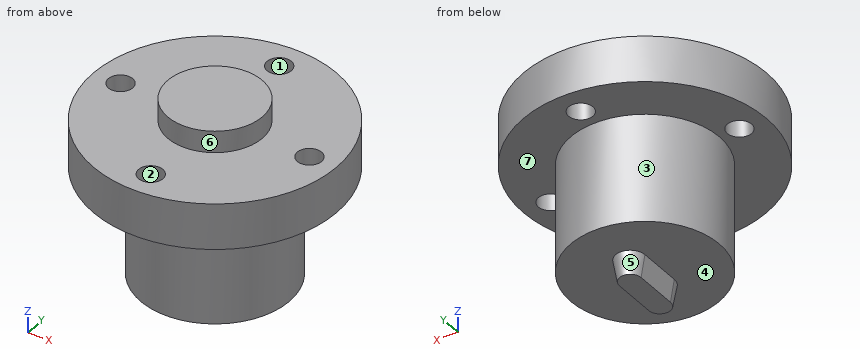
Autodesk Inventor part; units mm, degrees
ref_plane "YZ Plane" through (0, 0, 0) normal (1, 0, 0) x (0, 1, 0)
ref_plane "XZ Plane" through (0, 0, 0) normal (0, 1, 0) x (-1, 0, 0)
ref_plane "XY Plane" through (0, 0, 0) normal (0, 0, 1) x (1, 0, 0)
sketch "Esboço1" plane through (0, 0, 0) normal (0, 0, 1) x (1, 0, 0)
  circle A0 centre (0, 0) radius 27.5
  dimension "d0" = 55
extrude "Extrusão1" add sketch "Esboço1" along normal blind 40
sketch "Esboço2" plane through (0, 0, 40) normal (0, 0, 1) x (1, 0, 0)
  circle A0 centre (0, 0) radius 45
  dimension "d3" = 90
extrude "Extrusão2" add sketch "Esboço2" along normal blind 17
sketch "Esboço3" plane through (0, 0, 57) normal (0, 0, 1) x (1, 0, 0)
  circle A0 centre (35, 0) radius 4.5
  circle A1 centre (0, 35) radius 4.5
  circle A2 centre (-35, 0) radius 4.5
  circle A3 centre (0, -35) radius 4.5
  point P0 (0, 0)
  dimension "d7" = 9
  dimension "d8" = 35
  dimension "d11" = 360
extrude "Extrusão3" cut sketch "Esboço3" against normal blind 17.5
sketch "Esboço4" plane through (0, 0, 57) normal (0, 0, 1) x (1, 0, 0)
  circle A0 centre (0, 0) radius 27.5
  circle A1 centre (0, 0) radius 17.5
  dimension "d15" = 35
extrude "Extrusão4" add sketch "Esboço4" along normal blind 8 contours A1
sketch "Esboço6" plane through (0, 0, 0) normal (0, 0, -1) x (-1, 0, 0)
  line L0 (0, 8) -> (0, -8) construction
  line L1 (5.41, 8) -> (5.41, -8)
  line L2 (-5.41, -8) -> (-5.41, 8)
  arc A0 (5.41, 8) -> (-5.41, 8) centre (0, 8) ccw
  arc A1 (-5.41, -8) -> (5.41, -8) centre (0, -8) ccw
  point P0 (0, 0)
  point P1 (0, 0)
  dimension "d24" = 5.41
  dimension "d25" = 16
  dimension "d26" = 0
  dimension "d27" = 0
extrude "Extrusão5" add sketch "Esboço6" along normal blind 8 draft -10
properties part number "Matriz superior do Ferramental"
Verification items for the finished model (mm, model axes). Face numbers are marked on the shaded views. A direction names the side the tool comes from. Give positions to 0.01 mm unless a question says otherwise; leave off trailing zeros. Order: outer loops, then holes, each group sorted by start corner. A loop starts at its lowest first (then second) coordinate and runs counter-clockwise, first axis right, second up. Notation, with made-up numbers: M -22,56.25 L 0,56.25 A18 ccw 0,81.25 Z; hole C 67.5,-2.75 d9. An arc over 180 degrees is marked long. Return JSON: item names as keys, results as strings. Group by question number.
1) Section check B-B on x = 36. Record the cut outline in (y, z), and give its area (3 significant figures).
2) Section check C-C on x = 0. Record the cut outline in (y, z), and give its area (3 significant figures).
3) Go/stop test with flat-tipped pins: pin 1 Ø2 at (x, z) = (19.5, 9.5) entering from +Y; pin 2 Ø14.5 at (x, y) = (0, -35) entering from +Z; pin 3 Ø2 at (x, z) = (-17, 26.5) entering from -Y. Record where each tip stops, or that it passes through.
4) Section check D-D on z = 53. Record the cut outline in (x, y).
5) Section check A-A on y = 0. Record the cut outline in (x, z), and give its area (3 significant figures).
6) Mould release check, pull along Y, two halves, no side actions. Record for the marked faces 1, 2, 3 and 4: pulls with the +Y half, pulls with the -Y half, needs draft (parallel to the pull), parting line crosses it, or undercut.
7) Access from +Z, -Z, +X, -X, +Y, -Y to the whole of each face (thin tool, end or side, straight path). Record for the marked faces 5, 6 and 7.
8) Scan lines: line 1 (Y direction, x = 0, z = 49); line 2 (Z direction, x = 34, y = 23.5); line 3 (X direction, y = -2, z = 55). Record each from-to range of solid material in increasing order.
Answer block:
{
 "1": {"outline": "M -27,40 L -4.39,40 L -4.39,57 L -27,57 Z; M 4.39,40 L 27,40 L 27,57 L 4.39,57 Z", "area": "769 mm^2"},
 "2": {"outline": "M -45,40 L -39.5,40 L -39.5,57 L -45,57 Z; M -30.5,40 L -27.5,40 L -27.5,0 L -13.41,0 L -12,-8 L 12,-8 L 13.41,0 L 27.5,0 L 27.5,40 L 30.5,40 L 30.5,57 L 17.5,57 L 17.5,65 L -17.5,65 L -17.5,57 L -30.5,57 Z; M 39.5,40 L 45,40 L 45,57 L 39.5,57 Z", "area": "3,910 mm^2"},
 "3": {"pin 1": "stops at y = 20.35", "pin 2": "stops at z = 57", "pin 3": "stops at y = -22.37"},
 "4": {"outline": "C 0,0 d90; hole C -35,0 d9; hole C 0,-35 d9; hole C 0,35 d9; hole C 35,0 d9"},
 "5": {"outline": "M -45,40 L -39.5,40 L -39.5,57 L -45,57 Z; M -30.5,40 L -27.5,40 L -27.5,0 L -5.41,0 L -4,-8 L 4,-8 L 5.41,0 L 27.5,0 L 27.5,40 L 30.5,40 L 30.5,57 L 17.5,57 L 17.5,65 L -17.5,65 L -17.5,57 L -30.5,57 Z; M 39.5,40 L 45,40 L 45,57 L 39.5,57 Z", "area": "3,780 mm^2"},
 "6": {"face 1": "undercut", "face 2": "undercut", "face 3": "parting line crosses it", "face 4": "needs draft"},
 "7": {"face 5": "-Z, +Y", "face 6": "+Z", "face 7": "-Z"},
 "8": {"line 1": "y = -45 to -39.5, -30.5 to 30.5, 39.5 to 45", "line 2": "z = 40 to 57", "line 3": "x = -44.96 to -39.03, -30.97 to 30.97, 39.03 to 44.96"}
}
